Can you work these out from the model? Positions are in its coordinate system, mm. A direction names the side the tool comes from. Give positions to 0.01 mm unless a question says otherwise; leave off trailing zeros. Loops run counter-clockwise (first coordinate to the right, second up) from the corner with the lowest first, then second, coordinate; pieces in that order, holes last. Notation, with made-up numbers: (19, 74.25) -> (55, 74.25) arc R15 ccw to (55, 100.25) -> close; hole circle Ø6 at (33, 40). An arc over 180 degrees is marked (long way). Use CSV: the item, a comma, the result in double quotes.
Autodesk Inventor part; units mm, degrees
ref_plane "YZ Plane" through (0, 0, 0) normal (1, 0, 0) x (0, 1, 0)
ref_plane "XZ Plane" through (0, 0, 0) normal (0, 1, 0) x (-1, 0, 0)
ref_plane "XY Plane" through (0, 0, 0) normal (0, 0, 1) x (1, 0, 0)
sketch "Sketch1" plane through (0, 0, 0) normal (0, 0, 1) x (1, 0, 0)
  line L0 (0, 0) -> (150, 0)
  line L1 (150, 0) -> (150, 135)
  line L2 (150, 135) -> (0, 135)
  line L3 (0, 135) -> (0, 0)
  line L4 (0, 17.5) -> (-5, 17.5)
  line L5 (-5, 17.5) -> (-5, 82.5)
  line L6 (-5, 82.5) -> (0, 82.5)
  line L7 (0, 82.5) -> (0, 17.5)
  line L8 (75, 0) -> (75, 135) construction
  line L9 (150, 17.5) -> (155, 17.5)
  line L10 (155, 17.5) -> (155, 82.5)
  line L11 (155, 82.5) -> (150, 82.5)
  line L12 (150, 82.5) -> (150, 17.5)
  line L13 (45, 60) -> (105, 60)
  line L14 (105, 60) -> (105, 65)
  line L15 (105, 65) -> (45, 65)
  line L16 (45, 65) -> (45, 60)
  line L17 (0, 50) -> (150, 50) construction
  line L18 (45, 135) -> (105, 135)
  line L19 (105, 135) -> (105, 140)
  line L20 (105, 140) -> (45, 140)
  line L21 (45, 140) -> (45, 135)
  point P0 (150, 17.5)
  point P1 (150, 82.5)
  point P2 (0, 82.5)
  point P3 (10, 0)
  point P4 (45, 62.5)
  dimension "d0" = 150
  dimension "d1" = 135
  dimension "d2" = 5
  dimension "d3" = 65
  dimension "d6" = 60
  dimension "d7" = 5
  dimension "d14" = 30
  dimension "d30" = 60
  dimension "d31" = 5
  dimension "d32" = 45
  dimension "d58" = 52.5
  dimension "d59" = 60
extrude "Extrusion1" add sketch "Sketch1" along normal blind 5
sketch "Sketch2" plane through (0, 0, 5) normal (0, 0, 1) x (1, 0, 0)
  line L0 (150, 135) -> (0, 135)
  line L1 (0, 0) -> (150, 0)
  line L2 (0, 135) -> (0, 82.5)
  line L3 (0, 17.5) -> (0, 0)
  point P0 (75, 20)
  dimension "d24" = 20
  dimension "d29" = 75
hole "Hole1" at (75, 20, 5) direction (0, 0, -1) diameter 3 end through all
sketch "Sketch3" plane through (0, 0, 5) normal (0, 0, 1) x (1, 0, 0)
  line L0 (105, 140) -> (45, 140)
  line L1 (45, 140) -> (45, 135)
  line L2 (0, 135) -> (0, 82.5)
  point P0 (0, 0)
  point P1 (75, 120)
  dimension "d40" = 20
  dimension "d45" = 75
hole "Hole2" at (75, 120, 5) direction (0, 0, -1) diameter 3 end through all
sketch "Sketch4" plane through (0, 0, 5) normal (0, 0, 1) x (1, 0, 0)
  line L0 (-5, 82.5) -> (-5, 17.5)
  line L1 (0, 82.5) -> (-5, 82.5)
  line L2 (155, 82.5) -> (150, 82.5)
  line L3 (155, 17.5) -> (155, 82.5)
  point P0 (0, 0)
  point P1 (135, 50)
  point P2 (15, 50)
  point P3 (-5, 50)
  point P4 (-2.5, 82.5)
  dimension "d54" = 20
  dimension "d55" = 32.5
  dimension "d56" = 32.5
  dimension "d57" = 20
hole "Hole3" at (135, 50, 5) at (15, 50, 5) direction (0, 0, -1) diameter 3 end through all
properties part number "back" material "ABS Plastic"
(1) If we section it at D-D, the plane x = 38: Write out the boundary of the cut face in (y, z).
Answer sheet:
outline,"(0, 0) -> (135, 0) -> (135, 5) -> (0, 5) -> close"
(2) If I drill on L1, parallel to X at y = 50, z = 1.85; L2, parallel to Y at x = 75, z = 2.1; L3, parallel to Y at x = 79, z = 2.25, over which ranges is the centre line in solid material (lowest first)? Write a range as from..to.
Answer sheet:
L1,"x = -5..13.5, 16.5..133.5, 136.5..155"
L2,"y = 0..18.5, 21.5..60, 65..118.5, 121.5..140"
L3,"y = 0..60, 65..140"
(3) Which directions (+Z, -Z, +X, -X, +Y, -Y) give clear straight access to the entire face, cutting with the end or side of a thin tool? Please do faces 1 (the face through (-2, 17.5, 2)), 2 (the face through (45, 138, 2)), 3 (the face through (128, 135, 2)), 4 (the face through (75, 65, 2)), 5 (the face through (150, 9, 2)).
Answer sheet:
face 1,"+Z, -Z, -X, -Y"
face 2,"+Z, -Z, -X, +Y"
face 3,"+Z, -Z, +X, +Y"
face 4,"+Z, -Z"
face 5,"+Z, -Z, +X, -Y"
(4) We'd pull the mould along X, two halves only. Please class faces 6 (the face through (-5, 50, 2)), 7 (the face through (-3, 82.5, 2)), 8 (the face through (75, 60, 2)): released by +X, released by -X, zero draft, split by the parting line, or undercut.
Answer sheet:
face 6,"released by -X"
face 7,"zero draft"
face 8,"undercut"
(5) If we section it at C-C, the plane y = 96: Write out the boundary of the cut face in (x, z), then the cut area to 3 significant figures.
Answer sheet:
outline,"(0, 0) -> (150, 0) -> (150, 5) -> (0, 5) -> close"
area,"750 mm2"
(6) If we section it at A-A, the plane x = 99.5: Write out the boundary of the cut face in (y, z), then the cut area to 3 significant figures.
Answer sheet:
outline,"(0, 0) -> (60, 0) -> (60, 5) -> (0, 5) -> close; (65, 0) -> (140, 0) -> (140, 5) -> (65, 5) -> close"
area,"675 mm2"
(7) Will these pins go through, and if not, where does the flat tip stop? pin 1 Ø2 at (x, z) = (115, 4) entering from +Y; pin 2 Ø4 at (x, y) = (91, 25) entering from -Z; pin 3 Ø1.5 at (x, z) = (151.5, 1.5) entering from -Y; pin 4 Ø2.5 at (y, z) = (138.5, 2.5) entering from +X.
Answer sheet:
pin 1,"stops at y = 135"
pin 2,"stops at z = 0"
pin 3,"stops at y = 17.5"
pin 4,"stops at x = 105"
(8) If we section it at B-B, the plane z = 4: Write out the boundary of the cut face in (x, y).
Answer sheet:
outline,"(-5, 17.5) -> (0, 17.5) -> (0, 0) -> (150, 0) -> (150, 17.5) -> (155, 17.5) -> (155, 82.5) -> (150, 82.5) -> (150, 135) -> (105, 135) -> (105, 140) -> (45, 140) -> (45, 135) -> (0, 135) -> (0, 82.5) -> (-5, 82.5) -> close; hole circle Ø3 at (15, 50); hole (45, 60) -> (105, 60) -> (105, 65) -> (45, 65) -> close; hole circle Ø3 at (75, 20); hole circle Ø3 at (75, 120); hole circle Ø3 at (135, 50)"
